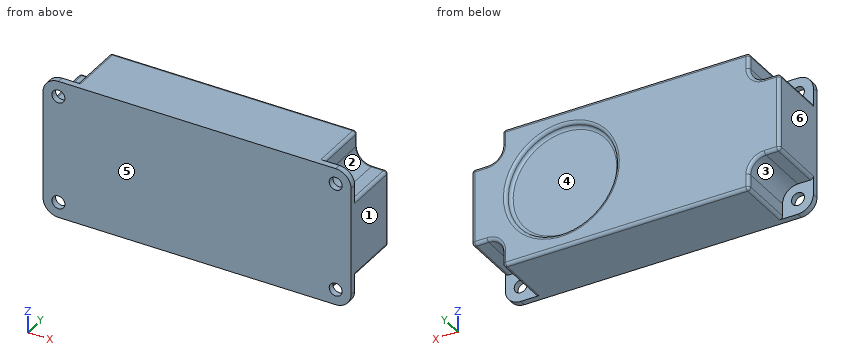
```python
from build123d import *

# Parameters (mm, degrees)
EXTRUDE_1_DEPTH     = 2
EXTRUDE_3_DEPTH     = 18.5
FILLET_1_R          = 1
SKETCH_4_R          = 17.821315346
CUT_EXTRUDE_1_DEPTH = 2
FILLET_2_R          = 1
SKETCH_5_R          = 2.1
CUT_EXTRUDE_2_DEPTH = 2


with BuildPart() as part:
    # 草图1 → 凸台-拉伸1 (new body)
    with BuildSketch(Plane(origin=(0, 0, 0), x_dir=(1, 0, 0), z_dir=(0, 1, 0))):
        with BuildLine():
            Line((-45, -22.5), (45, -22.5))
            ThreePointArc((45, -22.5), (48.535533906, -21.035533906), (50, -17.5))
            Line((50, -17.5), (50, 17.5))
            ThreePointArc((50, 17.5), (48.535533906, 21.035533906), (45, 22.5))
            Line((45, 22.5), (-45, 22.5))
            ThreePointArc((-45, 22.5), (-48.535533906, 21.035533906), (-50, 17.5))
            Line((-50, 17.5), (-50, -17.5))
            ThreePointArc((-50, -17.5), (-48.535533906, -21.035533906), (-45, -22.5))
        make_face()
    extrude(amount=EXTRUDE_1_DEPTH)

    # 草图2 → 凸台-拉伸3 (add)
    with BuildSketch(Plane(origin=(0, 2, 0), x_dir=(1, 0, 0), z_dir=(0, 1, 0))):
        with BuildLine():
            Line((-40, 22.5), (-40, 17.5))
            ThreePointArc((-40, 17.5), (-41.464466094, 13.964466094), (-45, 12.5))
            Line((-45, 12.5), (-50, 12.5))
            Line((-50, 12.5), (-50, -12.5))
            Line((-50, -12.5), (-45, -12.5))
            ThreePointArc((-45, -12.5), (-41.464466094, -13.964466094), (-40, -17.5))
            Line((-40, -17.5), (-40, -22.5))
            Line((-40, -22.5), (40, -22.5))
            Line((40, -22.5), (40, -17.5))
            ThreePointArc((40, -17.5), (41.464466094, -13.964466094), (45, -12.5))
            Line((45, -12.5), (50, -12.5))
            Line((50, -12.5), (50, 12.5))
            Line((50, 12.5), (45, 12.5))
            ThreePointArc((45, 12.5), (41.464466094, 13.964466094), (40, 17.5))
            Line((40, 17.5), (40, 22.5))
            Line((40, 22.5), (-40, 22.5))
        make_face()
    extrude(amount=EXTRUDE_3_DEPTH)

    # 圆角1
    fillet_1_edges = [part.edges().sort_by_distance(p)[0] for p in [
        (40, 11.25, -22.5),
        (-40, 11.25, -22.5),
        (-50, 11.25, -12.5),
        (-50, 11.25, 12.5),
        (-40, 11.25, 22.5),
        (40, 11.25, 22.5),
        (50, 11.25, 12.5),
        (50, 11.25, -12.5),
        (41.464466094, 20.5, -13.964466094),
        (40, 20.5, -20),
        (0, 20.5, -22.5),
        (-40, 20.5, -20),
        (-41.464466094, 20.5, -13.964466094),
        (-47.5, 20.5, -12.5),
        (-50, 20.5, 0),
        (-47.5, 20.5, 12.5),
        (-41.464466094, 20.5, 13.964466094),
        (-40, 20.5, 20),
        (0, 20.5, 22.5),
        (40, 20.5, 20),
        (41.464466094, 20.5, 13.964466094),
        (47.5, 20.5, 12.5),
        (50, 20.5, 0),
        (47.5, 20.5, -12.5),
    ]]
    fillet(fillet_1_edges, radius=FILLET_1_R)

    # 草图4 → 切除-拉伸1 (cut)
    with BuildSketch(Plane(origin=(0, 20.5, 0), x_dir=(1, 0, 0), z_dir=(0, 1, 0))):
        with Locations(Location((20.892434564, 0, 0), (0, 0, 270))):
            Circle(SKETCH_4_R)
    extrude(amount=-CUT_EXTRUDE_1_DEPTH, mode=Mode.SUBTRACT)

    # 圆角2
    fillet_2_edges = [part.edges().sort_by_distance(p)[0] for p in [
        (20.892434564, 18.5, -17.821315346),
        (20.892434564, 20.5, -17.821315346),
    ]]
    fillet(fillet_2_edges, radius=FILLET_2_R - 0.0001)  # a hair under: the kernel refuses the full size

    # 草图5 → 切除-拉伸2 (cut)
    with BuildSketch(Plane(origin=(0, 2, 0), x_dir=(1, 0, 0), z_dir=(0, 1, 0))):
        with Locations(Location((-45, 17.5, 0), (0, 0, 270))):
            Circle(SKETCH_5_R)
        with Locations(Location((45, 17.5, 0), (0, 0, 270))):
            Circle(SKETCH_5_R)
        with Locations(Location((45, -17.5, 0), (0, 0, 270))):
            Circle(SKETCH_5_R)
        with Locations(Location((-45, -17.5, 0), (0, 0, 270))):
            Circle(SKETCH_5_R)
    extrude(amount=-CUT_EXTRUDE_2_DEPTH, mode=Mode.SUBTRACT)


solid = part.part
```
Here's how the part is built. I have some questions about the finished solid (model axes, mm). Face numbers are marked on the shaded views. A direction names the side the tool comes from. Coordinates: 2 decimals unless noted, no trailing zeros. Write each loop counter-clockwise with the first axis right and the second up, starting at its lowest first coordinate (ties: lowest second). Pieces come first, ordered by that corner, then holes. Notation, with made-up numbers: M -15,81 L -9,81 A15 cw -9,108 Z; hole C 34.5,4.5 d2. An arc over 180 degrees is marked long. Answer as CSV lines item,"result". Start each with the question number.
Q1. For the marked faces 1, 2 and 3, which set-ups out of +Z, -Z, +X, -X, +Y, -Y let a thin tool reach every point of the face, with its end or its side?
Q2. Suppose I cut it at B-B, the plane y = 7. List the corners of the cut face in (x, z) for me, then the cut area to 3 significant figures.
Q3. Will these pins go through, and if not, where does the flat tip stop? pin 1 Ø2.5 at (x, z) = (45, 17.5) entering from -Y; pin 2 Ø9 at (x, z) = (47, 18) entering from +Y; pin 3 Ø17 at (x, z) = (18.5, -0.5) entering from +Y; pin 4 Ø2 at (y, z) = (10, 19.5) entering from +X.
Q4. If we mould it in two halves opening along X, with no side actions, what happens to the marked faces 4, 5 and 6? For each: pulls with the +X half, pulls with the -X half, needs draft (parallel to the pull), parting line crosses it, or undercut.
Q5. I need wall thicknesses on probe 1 along X at (y, z) = (19.5, 0); probe 2 along Y at (x, z) = (15, 8); probe 3 along X at (y, z) = (15, 18). Which ranges of each line are inside material? Lowest first, please. Write a range as [from, to].
Entries:
1,face 1,"+Z, -Z, +X, +Y, -Y"
1,face 2,"+Z, +X, +Y"
1,face 3,"-Z, -X, +Y"
2,outline,"M -50,-11.5 A1 ccw -49,-12.5 L -45,-12.5 A5 cw -40,-17.5 L -40,-21.5 A1 ccw -39,-22.5 L 39,-22.5 A1 ccw 40,-21.5 L 40,-17.5 A5 cw 45,-12.5 L 49,-12.5 A1 ccw 50,-11.5 L 50,11.5 A1 ccw 49,12.5 L 45,12.5 A5 cw 40,17.5 L 40,21.5 A1 ccw 39,22.5 L -39,22.5 A1 ccw -40,21.5 L -40,17.5 A5 cw -45,12.5 L -49,12.5 A1 ccw -50,11.5 Z"
2,area,"4,120 mm²"
3,pin 1,"passes through"
3,pin 2,"stops at y = 2"
3,pin 3,"stops at y = 18.5"
3,pin 4,"stops at x = 40"
4,face 4,"undercut"
4,face 5,"needs draft"
4,face 6,"pulls with the -X half"
5,probe 1,"x = [-50, 3.07], [38.71, 50]"
5,probe 2,"y = [0, 18.5]"
5,probe 3,"x = [-40, 40]"
